Part model, mm, in its own coordinate system. Face numbers are marked on the shaded views. A direction names the side the tool comes from. Round coordinates to 2 decimals unless told otherwise and drop trailing zeros. Loops run counter-clockwise (first coordinate to the right, second up) from the corner with the lowest first, then second, coordinate; pieces in that order, holes last. Notation, with made-up numbers: M -36,78.5 L -28,78.5 A16 cw -28,96.5 Z; hole C 35,23 d1. An arc over 180 degrees is marked long. Put each result on its own line as item: value. Start each with the question number.
1) Slice it at A-A on y = 0. Give the cut face in (x, z), then the cut area to 3 significant figures.
2) Slice it at B-B on x = -10.5. Give the cut face in (y, z), then the cut area to 3 significant figures.
3) Slice it at D-D on x = -28. Give the cut face in (y, z), then the cut area to 3 significant figures.
4) Slice it at C-C on z = 0. Give the cut face in (x, y), then the cut area to 3 significant figures.
5) Which spindle directions (+Z, -Z, +X, -X, +Y, -Y) get a long thin tool onto all of the face, cutting with end or side? Do the marked faces 1, 2 and 3. Say none if no direction does.
6) Probe line 1 along Y through (x, z) = (-4.5, 4.75); line 2 along X through (y, z) = (0.05, 0); line 3 along X through (y, z) = (2, 1.25). List the from-to ranges inside material, lowest first.
7) Drop flat-ended pins along their axis: pin 1 Ø3 at (y, z) = (3.5, -1) entering from -X; pin 2 Ø1 at (x, z) = (-4, 5) entering from +Y; pin 3 Ø6 at (x, z) = (-3.5, -2.5) entering from -Y; pin 4 Ø1.1 at (y, z) = (0, 5.5) entering from -X. Give the stop position or say it passes through.
8) Pull direction Z, two halves, no side cores. Call the marked faces 4, 5 and 6: +Z half, -Z half, draft (parallel to the pull), parting line (faces both ways), or undercut.
```python
from build123d import *

# Parameters (mm, degrees)
SKETCH2_R                      = 2.05
SKETCH2_R_2                    = 3
BOSS_EXTRUDE1_DEPTH            = 2.4
BOSS_EXTRUDE1_DEPTH_BACK       = 2.4
SKETCH10_W                     = 20.072017009
SKETCH10_H                     = 1
BOSS_EXTRUDE3_DEPTH            = 2.5
BOSS_EXTRUDE4_REACH            = 9.3
SKETCH11_W                     = 20.072017009
SKETCH11_H                     = 1
CUT_EXTRUDE1_REACH             = 31.685
CUT_EXTRUDE1_DIRECTION_2_REACH = 13.017
BOSS_EXTRUDE5_START            = -0.802964
SKETCH14_W                     = 6.607136291
SKETCH14_H                     = 1.4
BOSS_EXTRUDE5_DEPTH            = 1.802964
BOSS_EXTRUDE6_START            = -1
SKETCH16_W                     = 9.217702834
SKETCH16_H                     = 1.4
BOSS_EXTRUDE6_DEPTH            = 2
CHAMFER1_SIZE                  = 1.5
CHAMFER1_OF_MIRROR2_SIZE       = 1.5


with BuildPart() as part:
    # Sketch2 → Boss-Extrude1 (new body, two sides)
    with BuildSketch(Plane(origin=(0, 0, 0), x_dir=(1, 0, 0), z_dir=(0, 1, 0))) as boss_extrude1_sk:
        with BuildLine():
            Line((0.409273591, 4.678018553), (-29.476567352, 7.292690835))
            ThreePointArc((-29.476567352, 7.292690835), (-36, 1.571793945), (-30, -4.695887824))
            Line((-30, -4.695887824), (0, -4.695887824))
            ThreePointArc((0, -4.695887824), (4.691418379, -0.20483175), (0.409273591, 4.678018553))
        make_face()
        Circle(SKETCH2_R, mode=Mode.SUBTRACT)
        with Locations((-30, 1.309828287)):
            Circle(SKETCH2_R_2, mode=Mode.SUBTRACT)
        Polygon((-14.53364688, 5.985354694), (0.409273591, 4.678018553), (0.761927553, 6.678018553), align=None)
    extrude(amount=BOSS_EXTRUDE1_DEPTH)
    extrude(boss_extrude1_sk.sketch, amount=-BOSS_EXTRUDE1_DEPTH_BACK)

    # Sketch10 → Boss-Extrude3 (add)
    with BuildSketch(Plane(origin=(0, 2.4, 0), x_dir=(1, 0, 0), z_dir=(0, 1, 0))):
        with BuildLine():
            ThreePointArc((-25.883157303, 6.978308193), (-23.000951778, 1.004243242), (-26.392863709, -4.695887824))
            Line((-26.392863709, -4.695887824), (-6.3208467, -4.695887824))
            ThreePointArc((-6.3208467, -4.695887824), (-7.774768517, 1.247974345), (-4.53364688, 6.438207159))
            Line((-4.53364688, 6.438207159), (-14.53364688, 5.985354694))
            Line((-14.53364688, 5.985354694), (-25.883157303, 6.978308193))
        make_face()
        with Locations((-16.356855205, -5.195887824)):
            Rectangle(SKETCH10_W, SKETCH10_H)
    boss_extrude3 = extrude(amount=BOSS_EXTRUDE3_DEPTH)

    # Mirror1: Boss-Extrude3 across plane
    add(boss_extrude3.mirror(Plane.ZX))

    # Sketch11 → Boss-Extrude4 (add, up to next)
    with BuildSketch(Plane.XZ.offset(-2.4), mode=Mode.PRIVATE) as boss_extrude4_sk1:
        with Locations((-16.356855205, 5.195887824)):
            Rectangle(SKETCH11_W, SKETCH11_H)
    boss_extrude4_tool1 = extrude(boss_extrude4_sk1.sketch, amount=BOSS_EXTRUDE4_REACH, mode=Mode.PRIVATE) - part.part
    add(boss_extrude4_tool1.solids().sort_by_distance((-16.356855, 2.4, 5.195888))[0])

    # Sketch13 → Cut-Extrude1 (cut, up to next)
    with BuildSketch(Plane(origin=(-6.3208467, 0, 0), x_dir=(0, 0, -1), z_dir=(1, 0, 0)), mode=Mode.PRIVATE) as cut_extrude1_sk1:
        with BuildLine():
            Line((-4.695887824, -1), (-4.695887824, 1))
            ThreePointArc((-4.695887824, 1), (-3.695887824, 0), (-4.695887824, -1))
        make_face()
    cut_extrude1_tool1 = extrude(cut_extrude1_sk1.sketch, amount=-CUT_EXTRUDE1_REACH, mode=Mode.PRIVATE) & part.part
    add(cut_extrude1_tool1.solids().sort_by_distance((-6.320847, 0, 4.271475))[0], mode=Mode.SUBTRACT)

    # Sketch13 → Cut-Extrude1 direction 2 (cut, up to next)
    with BuildSketch(Plane(origin=(-6.3208467, 0, 0), x_dir=(0, 0, -1), z_dir=(1, 0, 0)), mode=Mode.PRIVATE) as cut_extrude1_direction_2_sk1:
        with BuildLine():
            Line((-4.695887824, -1), (-4.695887824, 1))
            ThreePointArc((-4.695887824, 1), (-3.695887824, 0), (-4.695887824, -1))
        make_face()
    cut_extrude1_direction_2_tool1 = extrude(cut_extrude1_direction_2_sk1.sketch, amount=CUT_EXTRUDE1_DIRECTION_2_REACH, mode=Mode.PRIVATE) & part.part
    add(cut_extrude1_direction_2_tool1.solids().sort_by_distance((-6.320847, 0, 4.271475))[0], mode=Mode.SUBTRACT)

    # Sketch14 → Boss-Extrude5 (add)
    with BuildSketch(Plane.XY.offset(4.695887824).offset(BOSS_EXTRUDE5_START)):
        with Locations((-29.696431854, -1.7)):
            Rectangle(SKETCH14_W, SKETCH14_H)
    boss_extrude5 = extrude(amount=BOSS_EXTRUDE5_DEPTH)

    # Sketch16 → Boss-Extrude6 (add)
    with BuildSketch(Plane.XY.offset(4.695887824).offset(BOSS_EXTRUDE6_START)):
        with Locations((-1.711995283, -1.7)):
            Rectangle(SKETCH16_W, SKETCH16_H)
    boss_extrude6 = extrude(amount=BOSS_EXTRUDE6_DEPTH)

    # Chamfer1
    chamfer1_edges = [part.edges().sort_by_distance(p)[0] for p in [
        (-33, -1.7, 5.695887824),
        (2.896856134, -1.7, 5.695887824),
    ]]
    chamfer(chamfer1_edges, length=CHAMFER1_SIZE)

    # Mirror2: Boss-Extrude5, Boss-Extrude6 across plane
    add(boss_extrude5.mirror(Plane.ZX))
    add(boss_extrude6.mirror(Plane.ZX))

    # Chamfer1 of Mirror2
    chamfer1_of_mirror2_edges = [part.edges().sort_by_distance(p)[0] for p in [
        (-33, 1.7, 5.695887824),
        (2.896856134, 1.7, 5.695887824),
    ]]
    chamfer(chamfer1_of_mirror2_edges, length=CHAMFER1_OF_MIRROR2_SIZE)


solid = part.part
```
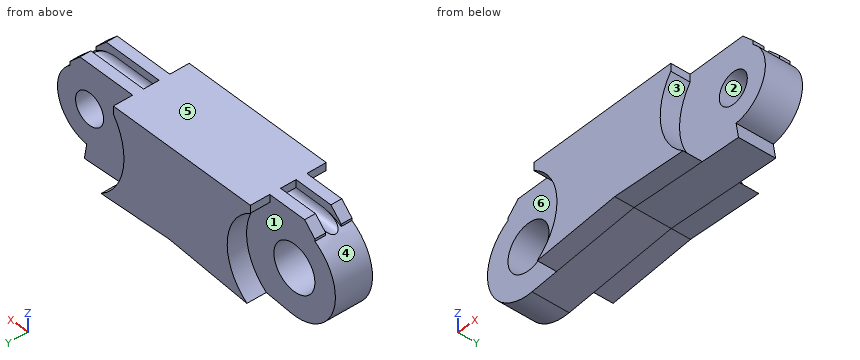
Recorded:
1. outline: M -33.32,3.7 A6.01 ccw -29.48,-7.29 L -14.53,-5.99 L 0.76,-6.68 L 0.41,-4.68 A4.7 ccw 2.9,3.7 Z; M -26.39,4.7 L -6.32,4.7 L -6.32,5.7 L -26.39,5.7 Z; hole C -30,-1.31 d6; hole C 0,0 d4.1
1. area: 372 mm2
2. outline: M -4.9,-6.17 L 4.9,-6.17 L 4.9,5.7 L -4.9,5.7 Z; hole M -1,4.7 A1 ccw 1,4.7 Z
2. area: 115 mm2
3. outline: M -2.4,-7.16 L 2.4,-7.16 L 2.4,-3.55 L -2.4,-3.55 Z; M -2.4,0.93 L 2.4,0.93 L 2.4,5.7 L 1,5.7 L 1,4.7 A1 cw -1,4.7 L -1,5.7 L -2.4,5.7 Z
3. area: 36.7 mm2
4. outline: M -35.86,-2.4 L -32.7,-2.4 L -32.7,2.4 L -35.86,2.4 Z; M -27.3,-2.4 L -23.12,-2.4 L -23.12,-4.9 L -7.87,-4.9 L -7.87,-2.4 L -2.05,-2.4 L -2.05,2.4 L -7.87,2.4 L -7.87,4.9 L -23.12,4.9 L -23.12,2.4 L -27.3,2.4 Z; M 2.05,-2.4 L 4.7,-2.4 L 4.7,2.4 L 2.05,2.4 Z
4. area: 225 mm2
5. face 1: -X, +Y
5. face 2: +Y, -Y
5. face 3: +X, -Y
6. line 1: y = -2.4 to -1, 1 to 2.4
6. line 2: x = -35.86 to -32.7, -27.3 to -2.05, 2.05 to 4.7
6. line 3: x = -35.43 to -31.56, -28.44 to -1.62, 1.62 to 4.53
7. pin 1: stops at x = -36.01
7. pin 2: stops at y = 2.4
7. pin 3: stops at y = -2.4
7. pin 4: stops at x = -26.39
8. face 4: parting line
8. face 5: +Z half
8. face 6: undercut
